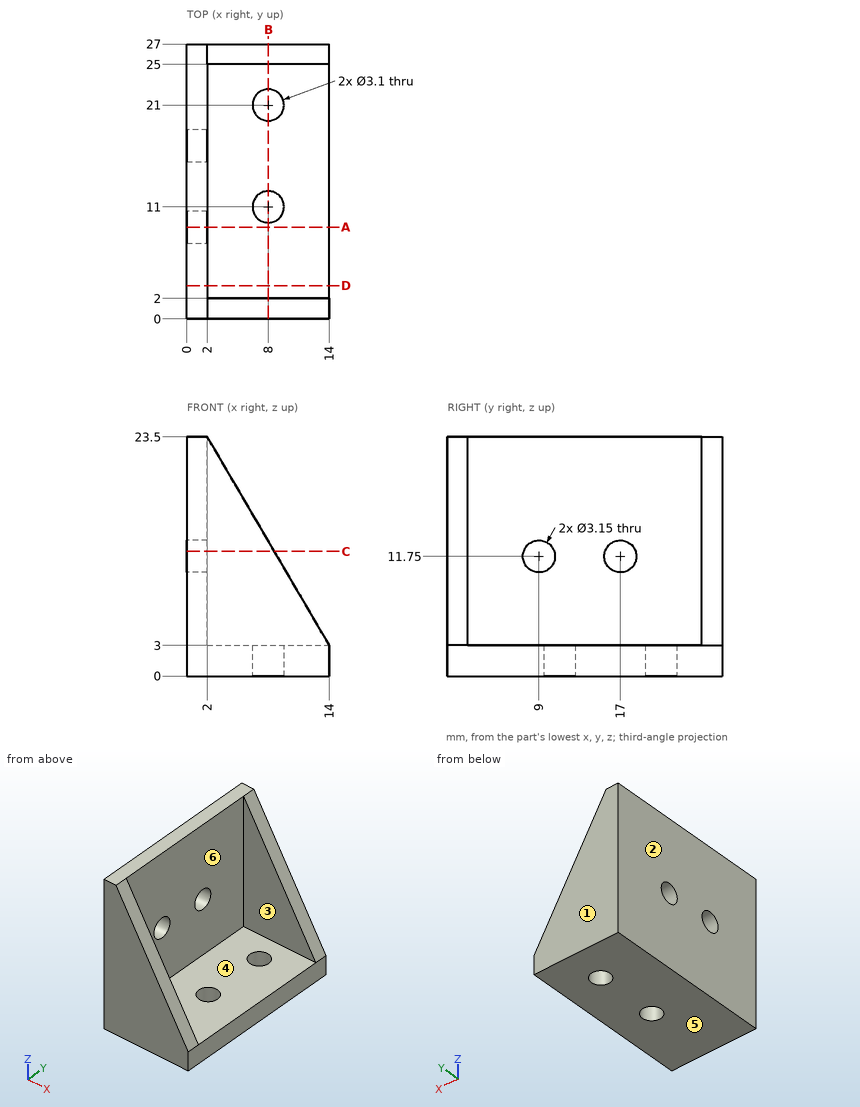
Drawing for the job (mm, zero at the part's lowest x, y, z). A direction names the side the tool comes from. Round coordinates to 2 decimals unless told otherwise and drop trailing zeros. Write each loop counter-clockwise with the first axis right and the second up, starting at its lowest first coordinate (ties: lowest second). Pieces come first, ordered by that corner, then holes. Notation, with made-up numbers: M 70.5,-38.75 L 98.5,-38.75 A12 ccw 98.5,-33.75 Z; hole C 59,49.5 d6. An arc over 180 degrees is marked long. Answer as a JSON object with one key per item and string values. Group by question number.
(1) Mould opens along Y. For the marked faces 1, 2, 3 and 4 say: pulls with the +Y half, pulls with the -Y half, needs draft (parallel to the pull), parting line crosses it, or undercut.
(2) Flat gauge pins, fed straight in: pin 1 (3.5 mm diameter, centred on y = 9, z = 11.75, fed in from -X); pin 2 (3 mm diameter, centred on x = 4.5, y = 15.5, fed in from +Z); pin 3 (3 mm diameter, centred on y = 8, z = 9.5, fed in from +X). Where does each tip first touch, or does it go through?
(3) Drill centre lines: L1, parallel to Y at x = 8, z = 0.8; L2, parallel to Y at x = 6.5, z = 10.5; L3, parallel to Y at x = 1.5, z = 10.5. Where is each one in solid material? Low to high.
(4) Cut at D-D (y = 3.25). Give the cut face in (x, z), and give its area (3 significant figures).
(5) Which spindle directions (+Z, -Z, +X, -X, +Y, -Y) get a long thin tool onto all of the face, cutting with end or side? Do the marked faces 5 and 6. Say none if no direction does.
(6) Cut at A-A (y = 9). Give the cut face in (x, z) (3 decimals), and give its area (3 significant figures).
(7) Cut at B-B (x = 8). Give the cut face in (y, z), and give its area (3 significant figures).
(8) Cut at C-C (z = 12.25). Give the cut face in (x, y), and give its area (3 significant figures).
Responses:
{
 "1": {"face 1": "pulls with the +Y half", "face 2": "needs draft", "face 3": "undercut", "face 4": "undercut"},
 "2": {"pin 1": "stops at x = 0", "pin 2": "stops at z = 3", "pin 3": "stops at x = 2"},
 "3": {"L1": "y = 0 to 9.45, 12.55 to 19.45, 22.55 to 27", "L2": "y = 0 to 2, 25 to 27", "L3": "y = 0 to 8.04, 9.96 to 16.04, 17.96 to 27"},
 "4": {"outline": "M 0,0 L 14,0 L 14,3 L 2,3 L 2,23.5 L 0,23.5 Z", "area": "83.0 mm2"},
 "5": {"face 5": "-Z, +X, -X, +Y, -Y", "face 6": "+Z, +X"},
 "6": {"outline": "M 0,0 L 14,0 L 14,3 L 2,3 L 2,10.175 L 0,10.175 Z; M 0,13.325 L 2,13.325 L 2,23.5 L 0,23.5 Z", "area": "76.7 mm2"},
 "7": {"outline": "M 0,0 L 9.45,0 L 9.45,3 L 2,3 L 2,13.25 L 0,13.25 Z; M 12.55,0 L 19.45,0 L 19.45,3 L 12.55,3 Z; M 22.55,0 L 27,0 L 27,13.25 L 25,13.25 L 25,3 L 22.55,3 Z", "area": "103 mm2"},
 "8": {"outline": "M 0,0 L 8.59,0 L 8.59,2 L 2,2 L 2,7.51 L 0,7.51 Z; M 0,10.49 L 2,10.49 L 2,15.51 L 0,15.51 Z; M 0,18.49 L 2,18.49 L 2,25 L 8.59,25 L 8.59,27 L 0,27 Z", "area": "68.4 mm2"}
}
